Design review of the part built by this model. Coordinates are the model's own, in mm. Coordinates: 2 decimals unless noted, no trailing zeros. Write each loop counter-clockwise with the first axis right and the second up, starting at its lowest first coordinate (ties: lowest second). Pieces come first, ordered by that corner, then holes. Notation, with made-up numbers: M 13.25,65.25 L 20.25,65.25 A25 cw 20.25,81.25 Z; hole C -24.5,20.5 d5. An arc over 180 degrees is marked long. Write each question's results on one line, items separated by ' | '. Start each with the question number.
```python
from build123d import *

# Parameters (mm, degrees)
SKETCH1_R           = 2.25
BOSS_EXTRUDE1_DEPTH = 5
SKETCH2_W           = 48.1
SKETCH2_H           = 93.7
SKETCH2_R           = 2.25
BOSS_EXTRUDE2_DEPTH = 5
BOSS_EXTRUDE3_START = -5
SKETCH3_R           = 2.25
BOSS_EXTRUDE3_DEPTH = 5


with BuildPart() as part:
    # Sketch1 → Boss-Extrude1 (new body)
    with BuildSketch(Plane.XY):
        with BuildLine():
            Line((-52.1605695, -11.804270746), (-52.1605695, 11.984503151))
            ThreePointArc((-52.1605695, 11.984503151), (-50.416314539, 17.627434468), (-45.792034729, 21.301823597))
            Line((-45.792034729, 21.301823597), (27.8394305, 50))
            Line((27.8394305, 50), (27.8394305, -43.667964744))
            Line((27.8394305, -43.667964744), (-45.084961564, -21.367111906))
            ThreePointArc((-45.084961564, -21.367111906), (-50.199348034, -17.752214901), (-52.1605695, -11.804270746))
        make_face()
        with Locations((-42.523814383, 0)):
            Circle(SKETCH1_R, mode=Mode.SUBTRACT)
        with Locations((-21.523814383, 0)):
            Circle(SKETCH1_R, mode=Mode.SUBTRACT)
        with Locations((8.476185617, 0)):
            Circle(SKETCH1_R, mode=Mode.SUBTRACT)
    extrude(amount=BOSS_EXTRUDE1_DEPTH)

    # Sketch2 → Boss-Extrude2 (add)
    with BuildSketch(Plane(origin=(27.8394305, 0, 0), x_dir=(0, 0, -1), z_dir=(1, 0, 0))):
        with Locations((-24.05, 3.15)):
            Rectangle(SKETCH2_W, SKETCH2_H)
        with Locations(Location((-35.6, 30, 0), (0, 0, 90))):
            Circle(SKETCH2_R, mode=Mode.SUBTRACT)
        with Locations(Location((-12.5, 30, 0), (0, 0, 90))):
            Circle(SKETCH2_R, mode=Mode.SUBTRACT)
        with Locations(Location((-35.6, -23.7, 0), (0, 0, 90))):
            Circle(SKETCH2_R, mode=Mode.SUBTRACT)
        with Locations(Location((-12.5, -23.7, 0), (0, 0, 90))):
            Circle(SKETCH2_R, mode=Mode.SUBTRACT)
    extrude(amount=BOSS_EXTRUDE2_DEPTH)

    # Sketch3 → Boss-Extrude3 (add)
    with BuildSketch(Plane.XY.offset(48.1).offset(BOSS_EXTRUDE3_START)):
        with BuildLine():
            Line((27.8394305, 50), (-45.792034729, 21.301823597))
            ThreePointArc((-45.792034729, 21.301823597), (-50.416314539, 17.627434468), (-52.1605695, 11.984503151))
            Line((-52.1605695, 11.984503151), (-52.1605695, -11.804270746))
            ThreePointArc((-52.1605695, -11.804270746), (-50.199348034, -17.752214901), (-45.084961564, -21.367111906))
            Line((-45.084961564, -21.367111906), (27.8394305, -43.7))
            Line((27.8394305, -43.7), (27.8394305, 50))
        make_face()
        with Locations((-21.523814383, 0)):
            Circle(SKETCH3_R, mode=Mode.SUBTRACT)
        with Locations((-42.523814383, 0)):
            Circle(SKETCH3_R, mode=Mode.SUBTRACT)
        with Locations((8.476185617, 0)):
            Circle(SKETCH3_R, mode=Mode.SUBTRACT)
    extrude(amount=BOSS_EXTRUDE3_DEPTH)


solid = part.part
```
Item 1: Insertion check: pin 1 Ø5 at (x, z) = (-25.5, 41) entering from -Y; pin 2 Ø13 at (y, z) = (10.5, 31.5) entering from -X; pin 3 Ø4 at (x, y) = (-42.52, 0) entering from -Z; pin 4 Ø10 at (x, z) = (0.5, 6.5) entering from +Y. Each pin has a flat end and moves straight along its axis. Give the tip position at first contact, or say it passes through.
Item 2: We need section B-B on z = 35.6. State the section outline as (x, y) points.
Item 3: Wall thickness on L1, parallel to Z at x = 30.3, y = -23.7; L2, parallel to Z at x = 14, y = -8.5; L3, parallel to Y at x = 29, z = 35: over which ranges is each line inside the solid? List them lowest first.
Item 4: We need section A-A on y = 0. Count the separate pieces of the cut face and the enclosed holes in it, then the cut area to 4 significant figures.
Item 5: Draft analysis for pull direction Z (two halves, no side actions). For faces 1 (the flat face through (30, 50, 24)), 2 (the flat face through (-3, 4, 5)), 3 (the flat face through (-4, 4, 43.1)), state which applies: released by +Z, released by -Z, zero draft, split by the parting line, or undercut.
Item 6: We need section D-D on z = 44.5. State the section outline as (x, y) points.
Item 7: We need section C-C on x = -33.5. State the section outline as (y, z) points.
Answer:
1) pin 1: stops at y = -27.78 | pin 2: stops at x = 27.84 | pin 3: passes through | pin 4: stops at y = 41.2
2) outline: M 27.84,-43.7 L 32.84,-43.7 L 32.84,-25.95 L 27.84,-25.95 Z; M 27.84,-21.45 L 32.84,-21.45 L 32.84,27.75 L 27.84,27.75 Z; M 27.84,32.25 L 32.84,32.25 L 32.84,50 L 27.84,50 Z
3) L1: z = 0 to 10.25, 14.75 to 33.35, 37.85 to 48.1 | L2: z = 0 to 5, 43.1 to 48.1 | L3: y = -43.7 to -25.87, -21.53 to 27.83, 32.17 to 50
4) separate pieces: 7 | enclosed holes: 0 | area: 905.5 mm^2
5) face 1: zero draft | face 2: undercut | face 3: undercut
6) outline: M -52.16,-11.8 A10 ccw -45.08,-21.37 L 27.84,-43.7 L 32.84,-43.7 L 32.84,50 L 27.84,50 L -45.79,21.3 A10 ccw -52.16,11.98 Z; hole C -42.52,0 d4.5; hole C -21.52,0 d4.5; hole C 8.48,0 d4.5
7) outline: M -24.91,0 L 26.09,0 L 26.09,5 L -24.91,5 Z; M -24.91,43.1 L 26.09,43.1 L 26.09,48.1 L -24.91,48.1 Z
